```python
from build123d import *

# Parameters (mm, degrees)
SKETCH2_W           = 29
SKETCH2_H           = 50
SKETCH2_R           = 2.425
SKETCH2_W_2         = 22
SKETCH2_H_2         = 25
BOSS_EXTRUDE1_DEPTH = 22.5
SKETCH3_R           = 1.755
SKETCH3_R_2         = 2.9
CUT_EXTRUDE1_DEPTH  = 30


with BuildPart() as part:
    # Sketch2 → Boss-Extrude1 (new body)
    with BuildSketch(Plane.XY):
        Rectangle(SKETCH2_W, SKETCH2_H)
        with Locations((0, 19.9)):
            Circle(SKETCH2_R, mode=Mode.SUBTRACT)
        with Locations((0, -19.9)):
            Circle(SKETCH2_R, mode=Mode.SUBTRACT)
        Rectangle(SKETCH2_W_2, SKETCH2_H_2, mode=Mode.SUBTRACT)
    extrude(amount=BOSS_EXTRUDE1_DEPTH)

    # Sketch3 → Cut-Extrude1 (cut)
    with BuildSketch(Plane(origin=(14.5, 0, 0), x_dir=(0, 0, -1), z_dir=(1, 0, 0))):
        with Locations((-5, 15)):
            Circle(SKETCH3_R)
        with Locations((-5, -15)):
            Circle(SKETCH3_R)
        with Locations((-15, 0)):
            Circle(SKETCH3_R_2)
    extrude(amount=-CUT_EXTRUDE1_DEPTH, mode=Mode.SUBTRACT)


solid = part.part
```
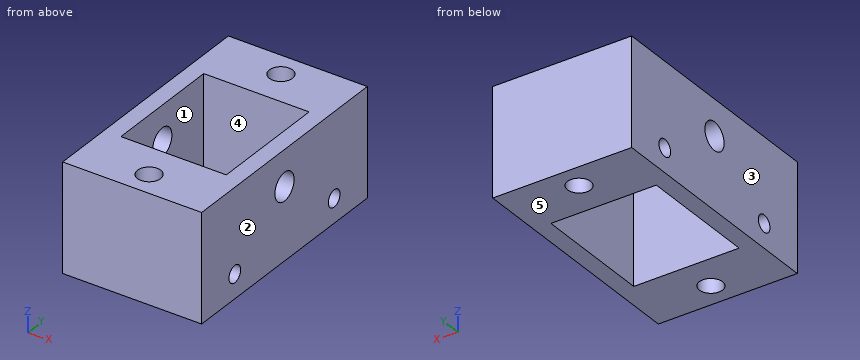
Part model, mm, in its own coordinate system. Face numbers are marked on the shaded views. A direction names the side the tool comes from. Round coordinates to 2 decimals unless told otherwise and drop trailing zeros. Write each loop counter-clockwise with the first axis right and the second up, starting at its lowest first coordinate (ties: lowest second). Pieces come first, ordered by that corner, then holes.
Item 1: Two-plate mould, pull along X, no slides. Class the marked faces 3, 4 and 5: +X half, -X half, draft (parallel to the pull), parting line (faces both ways), or undercut.
Results:
face 3: -X half
face 4: undercut
face 5: draft
Item 2: Cut at A-A, the plane x = -3. Give the cut face in (y, z) (3 decimals).
Results:
outline: (-25, 0) - (-12.5, 0) - (-12.5, 22.5) - (-25, 22.5) - close; (12.5, 0) - (25, 0) - (25, 22.5) - (12.5, 22.5) - close; hole circle Ø3.51 at (-15, 5); hole circle Ø3.51 at (15, 5)
Item 3: Cut at B-B, the plane z = 15. Give the cut face in (x, y) (3 decimals).
Results:
outline: (-14.5, -25) - (14.5, -25) - (14.5, -2.9) - (11, -2.9) - (11, -12.5) - (-11, -12.5) - (-11, -2.9) - (-14.5, -2.9) - close; (-14.5, 2.9) - (-11, 2.9) - (-11, 12.5) - (11, 12.5) - (11, 2.9) - (14.5, 2.9) - (14.5, 25) - (-14.5, 25) - close; hole circle Ø4.85 at (0, -19.9); hole circle Ø4.85 at (0, 19.9)
Item 4: Cut at D-D, the plane x = 0. Give the cut face in (y, z) (3 decimals).
Results:
outline: (-25, 0) - (-22.325, 0) - (-22.325, 22.5) - (-25, 22.5) - close; (-17.475, 0) - (-12.5, 0) - (-12.5, 22.5) - (-17.475, 22.5) - close; (12.5, 0) - (17.475, 0) - (17.475, 22.5) - (12.5, 22.5) - close; (22.325, 0) - (25, 0) - (25, 22.5) - (22.325, 22.5) - close; hole circle Ø3.51 at (-15, 5); hole circle Ø3.51 at (15, 5)
Item 5: Probe L1, parallel to Y at x = 8.25, z = 5 (3 decimals); L2, parallel to Y at x = 0, z = 14.25 (3 decimals); L3, parallel to X at y = 2, z = 5.25. List the from-to ranges inside material, lowest first.
Results:
L1: y = -25 to -16.755, -13.245 to -12.5, 12.5 to 13.245, 16.755 to 25
L2: y = -25 to -22.325, -17.475 to -12.5, 12.5 to 17.475, 22.325 to 25
L3: x = -14.5 to -11, 11 to 14.5
Item 6: Which spindle directions (+Z, -Z, +X, -X, +Y, -Y) get a long thin tool onto all of the face, cutting with end or side? Do the marked faces 1 and 2. Say none if no direction does.
Results:
face 1: +Z, -Z
face 2: +Z, -Z, +X, +Y, -Y
Item 7: Cut at C-C, the plane z = 5. Give the cut face in (x, y) (3 decimals).
Results:
outline: (-14.5, -25) - (14.5, -25) - (14.5, -16.755) - (-14.5, -16.755) - close; (-14.5, -13.245) - (14.5, -13.245) - (14.5, 13.245) - (-14.5, 13.245) - close; (-14.5, 16.755) - (14.5, 16.755) - (14.5, 25) - (-14.5, 25) - close; hole (-11, -12.5) - (11, -12.5) - (11, 12.5) - (-11, 12.5) - close; hole circle Ø4.85 at (0, -19.9); hole circle Ø4.85 at (0, 19.9)
